Here's the drawing with two shaded views (mm, measured from the low corner). I have some questions. A direction names the side the tool comes from. Round coordinates to 2 decimals unless told otherwise and drop trailing zeros. Order: outer loops, then holes, each group sorted by start corner. A loop starts at its lowest first (then second) coordinate and runs counter-clockwise, first axis right, second up. Notation, with made-up numbers: (-18, 42.25) -> (-7, 42.25) arc R19 cw to (-7, 66.25) -> close; hole circle Ø5 at (-7, 13). An arc over 180 degrees is marked (long way). Put each result on its own line as item: value. Start each with the question number.
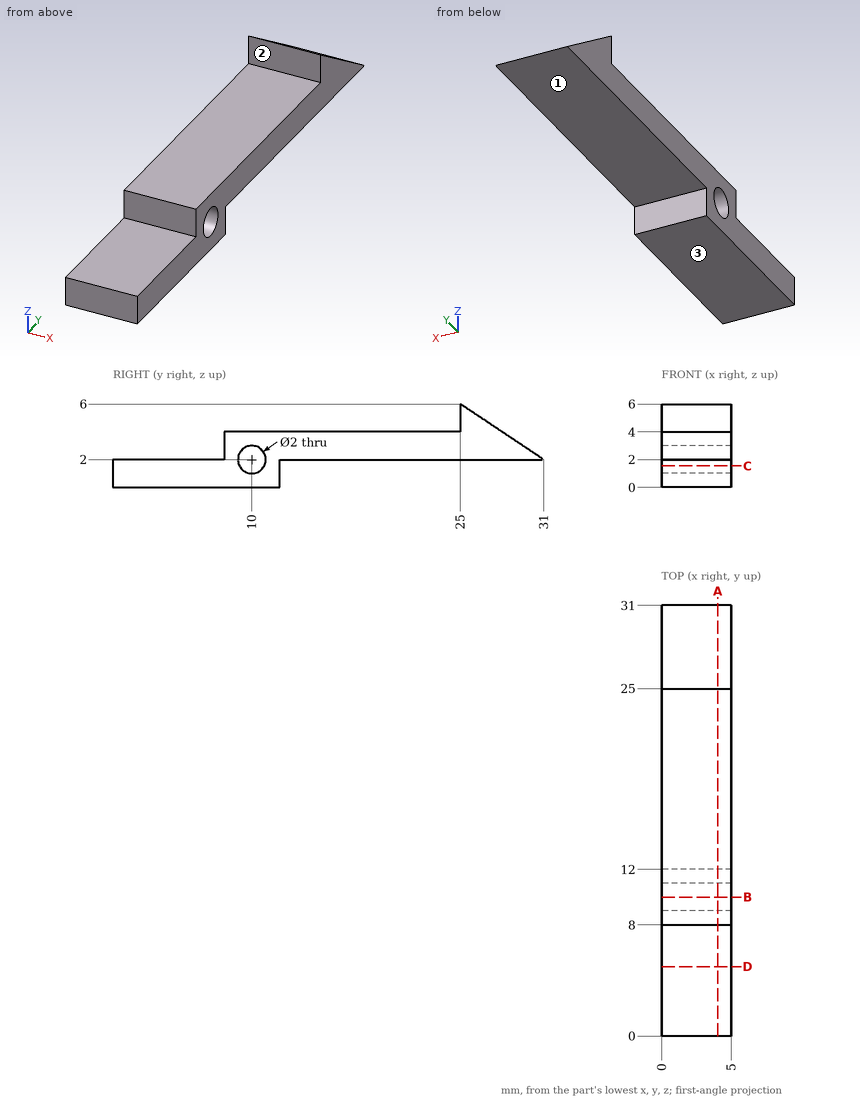
1. If we section it at A-A, the plane x = 4.05: Please give me the cut outline in (y, z), then the cut area to 3 significant figures.
2. I need wall thicknesses on L1, parallel to Z at x = 2.6, y = 23; L2, parallel to Y at x = 1.35, z = 0.9; L3, parallel to Y at x = 0.95, z = 2.2. Which ranges of each line are inside material? Lowest first, please.
3. If we section it at C-C, the plane z = 1.55: Please give me the cut outline in (x, y).
4. Which directions (+Z, -Z, +X, -X, +Y, -Y) give clear straight access to the entire face, cutting with the end or side of a thin tool? Please do the marked faces 1, 2 and 3.
5. For pin 1 Ø1.5 at (x, y) = (1.5, 20.5) entering from +Z; pin 2 Ø0.6 at (x, z) = (2.5, 5) entering from -Y; pin 3 Ø2.5 at (x, y) = (3, 4.5) entering from +Z, each with a flat end and sliding along its axis, tell me the tip position at first contact or that it passes through.
6. If we section it at B-B, the plane y = 10: Please give me the cut outline in (x, z), then the cut area to 3 significant figures.
7. If we section it at D-D, the plane y = 5: Please give me the cut outline in (x, z).
Results below:
1. outline: (0, 0) -> (12, 0) -> (12, 2) -> (31, 2) -> (25, 6) -> (25, 4) -> (8, 4) -> (8, 2) -> (0, 2) -> close; hole circle Ø2 at (10, 2)
1. area: 66.9 mm2
2. L1: 2 to 4
2. L2: 0 to 12
2. L3: 8 to 9.02, 10.98 to 30.7
3. outline: (0, 0) -> (5, 0) -> (5, 9.11) -> (0, 9.11) -> close; (0, 10.89) -> (5, 10.89) -> (5, 12) -> (0, 12) -> close
4. face 1: -Z, +X, -X, +Y
4. face 2: +Z, +X, -X, -Y
4. face 3: -Z, +X, -X, +Y, -Y
5. pin 1: z = 4
5. pin 2: y = 25
5. pin 3: z = 2
6. outline: (0, 0) -> (5, 0) -> (5, 1) -> (0, 1) -> close; (0, 3) -> (5, 3) -> (5, 4) -> (0, 4) -> close
6. area: 10.0 mm2
7. outline: (0, 0) -> (5, 0) -> (5, 2) -> (0, 2) -> close
